For this review, take the finished solid that the model builds, in its own axes (mm). Face numbers are marked on the shaded views. A direction names the side the tool comes from. Coordinates: 2 decimals unless noted, no trailing zeros. Loops run counter-clockwise (first coordinate to the right, second up) from the corner with the lowest first, then second, coordinate; pieces in that order, holes last. Notation, with made-up numbers: (26.5, 60) - (49.5, 60) arc R18 ccw to (49.5, 78) - close; hole circle Ø6 at (33, 27). An arc over 180 degrees is marked (long way). Answer as a JSON object with one key per item and string values. Group by question number.
Item 1: We need section A-A (y = 0). State how many separate pieces and enclosed holes the cut face has, then the cut area to 3 significant figures.
Item 2: We need section B-B (z = -0.5). Give the boundary of the cut face in (x, y).
Item 3: Tool access review of the marked faces 4, 5, 6, 7 and 8: name each direction out of +Z, -Z, +X, -X, +Y, -Y from which nothing blocks a thin tool from reaching the whole face with its end or side.
Item 4: To check wall thickness, follow line 1 (Y direction, x = -49, z = -17.5); line 2 (X direction, y = 4.5, z = -17); line 3 (X direction, y = 4.5, z = -19). State the ranges of each line that lie inside material, in increasing order.
Item 5: Mouldability with a two-part tool opening along X and no side actions: class the marked faces 1, 2 and 3 as released by +X, released by -X, zero draft, split by the parting line, or undercut.
Item 6: Clearance check with flat-ended pins moving along their axes: pin 1 (1.5 mm diameter, centred on x = 30, y = -7, fed in from +Z); pin 2 (2 mm diameter, centred on y = 7.5, z = 1.5, fed in from +X); pin 3 (14 mm diameter, centred on x = 0, z = 26.14, fed in from +Y); pin 4 (8 mm diameter, centred on x = 46.67, y = 0, fed in from -Z). State where each tip first meets the part, or that it passes through.
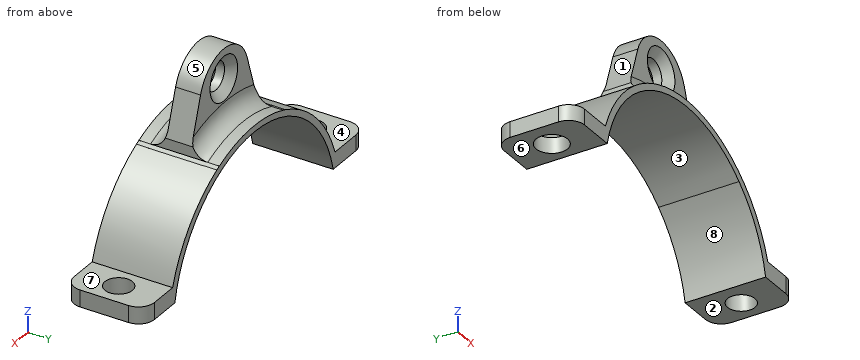
from build123d import *

# Parameters (mm, degrees)
F1_DEPTH  = 3.943235
F3_DEPTH  = 12.7
F4_R      = 5.08
F6_DEPTH  = 12.7
F7_W      = 17.78
F7_H      = 5.3086
F8_DEPTH  = 12.7
F9_DEPTH  = 8.66714
F10_DEPTH = 9.47498
F12_DEPTH = 12.7
F13_DEPTH = 12.7
F14_R     = 4.3985303862
F15_DEPTH = 53.72973
F16_SIZE  = 2.54
F17_SIZE  = 2.54
F18_R     = 5.08
F19_R     = 4.960906564
F19_R_2   = 4.3415616657
F20_DEPTH = 23.4886
F22_DEPTH = 18.208115
F24_DEPTH = 12.7
F26_DEPTH = 20.13737


with BuildPart() as f1:
    # F0 (on Front) → F1 (new body, symmetric)
    with BuildSketch(Plane.XZ):
        with BuildLine():
            Line((-11.7292143404, 26.9492678344), (-17.5938215107, 9.0761780739))
            ThreePointArc((-17.5938215107, 9.0761780739), (0, 11.6662775846), (17.5938215107, 9.0761780739))
            Line((17.5938215107, 9.0761780739), (11.7292143404, 26.9492678344))
            ThreePointArc((11.7292143404, 26.9492678344), (0, 35.4451148535), (-11.7292143404, 26.9492678344))
        make_face()
    extrude(amount=F1_DEPTH, both=True)

    # F2 (on Front) → F3 (join, symmetric)
    with BuildSketch(Plane.XZ):
        with BuildLine():
            Line((36.3047122955, -16.6163872927), (39.93518278, -16.6163872927))
            ThreePointArc((39.93518278, -16.6163872927), (-0.7137528874, 13.5858944169), (-42.1693213284, -15.4993189499))
            Line((-42.1693213284, -15.4993189499), (-39.0973836184, -15.7785862684))
            ThreePointArc((-39.0973836184, -15.7785862684), (-1.101821027, 10.3088316272), (36.3047122955, -16.6163872927))
        make_face()
    extrude(amount=F3_DEPTH, both=True)

    # F4
    f4_edges = [f1.edges().sort_by_distance(p)[0] for p in [
        (0.356921, -3.943235, 13.558065),
        (0.356921, 3.943235, 13.558065),
    ]]
    fillet(f4_edges, radius=F4_R)

    # F5 (on Front) → F6 (join, symmetric)
    with BuildSketch(Plane.XZ):
        Polygon((-39.8543514311, -20.1193168759), (-39.659883827, -15.2054578066), (-57.6343514311, -15.2054578066), (-57.6343514311, -20.1193168759), align=None)
    extrude(amount=F6_DEPTH, both=True)

    # F7 (on Front) → F8 (join, symmetric)
    with BuildSketch(Plane.XZ):
        with Locations((45.0512229579, -18.7627813943)):
            Rectangle(F7_W, F7_H)
    extrude(amount=F8_DEPTH, both=True)

    # F5 (on Front) → F9 (join)
    with BuildSketch(Plane.XZ):
        Polygon((-39.8543514311, -20.1193168759), (-39.659883827, -15.2054578066), (-57.6343514311, -15.2054578066), (-57.6343514311, -20.1193168759), align=None)
    extrude(amount=F9_DEPTH)

    # F7 (on Front) → F10 (join)
    with BuildSketch(Plane.XZ):
        with Locations((45.0512229579, -18.7627813943)):
            Rectangle(F7_W, F7_H)
    extrude(amount=F10_DEPTH)

    # F11 (on Front) → F12 (cut, symmetric)
    with BuildSketch(Plane.XZ):
        with BuildLine():
            ThreePointArc((-40.8051013947, -20.0025010854), (-1.7400987678, -54.2430909447), (38.6715009809, -21.6027013958))
            ThreePointArc((38.6715009809, -21.6027013958), (-0.4185114947, 11.3957328504), (-40.8051013947, -20.0025010854))
        make_face()
    extrude(amount=F12_DEPTH, both=True, mode=Mode.SUBTRACT)

    # F11 (on Front) → F13 (cut, symmetric)
    with BuildSketch(Plane.XZ):
        with BuildLine():
            ThreePointArc((-40.8051013947, -20.0025010854), (-1.7400987678, -54.2430909447), (38.6715009809, -21.6027013958))
            ThreePointArc((38.6715009809, -21.6027013958), (-0.4185114947, 11.3957328504), (-40.8051013947, -20.0025010854))
        make_face()
    extrude(amount=F13_DEPTH, both=True, mode=Mode.SUBTRACT)

    # F14 (on face) → F15 (cut, symmetric)
    with BuildSketch(Plane.XZ.offset(3.943235)):
        with Locations((0, 26.1365994811)):
            Circle(F14_R)
    extrude(amount=F15_DEPTH, both=True, mode=Mode.SUBTRACT)

    # F16
    f16_edges = [f1.edges().sort_by_distance(p)[0] for p in [
        (-4.39853, -3.943235, 26.136599),
    ]]
    chamfer(f16_edges, length=F16_SIZE)

    # F17
    f17_edges = [f1.edges().sort_by_distance(p)[0] for p in [
        (-4.39853, 3.943235, 26.136599),
    ]]
    chamfer(f17_edges, length=F17_SIZE)

    # F18
    f18_edges = [f1.edges().sort_by_distance(p)[0] for p in [
        (53.941223, 12.7, -18.762781),
        (53.941223, -12.7, -18.762781),
        (-57.634351, 12.7, -17.662387),
        (-57.634351, -12.7, -17.662387),
    ]]
    fillet(f18_edges, radius=F18_R)

    # F19 (on face) → F20 (cut)
    with BuildSketch(Plane.XY.offset(-15.2054578066)):
        with Locations((-48.8061010838, 0)):
            Circle(F19_R)
        with Locations((46.67250067, 0)):
            Circle(F19_R_2)
    extrude(amount=-F20_DEPTH, mode=Mode.SUBTRACT)

    # F21 (on Front) → F22 (cut, symmetric)
    with BuildSketch(Plane.XZ):
        with BuildLine():
            Line((-41.792165488, -23.9205155522), (39.0426814556, -25.9368028492))
            ThreePointArc((39.0426814556, -25.9368028492), (-0.4636625416, 11.5973705937), (-41.792165488, -23.9205155522))
        make_face()
    extrude(amount=F22_DEPTH, both=True, mode=Mode.SUBTRACT)

    # F23 (on Front) → F24 (cut, symmetric)
    with BuildSketch(Plane.XZ):
        Polygon((-17.0922335237, 10.6045696884), (-15.9068014473, 11.0168391839), (-15.9068014473, 14.8834753782), align=None)
    extrude(amount=F24_DEPTH, both=True, mode=Mode.SUBTRACT)

    # F25 (on Front) → F26 (cut, symmetric)
    with BuildSketch(Plane.XZ):
        Polygon((17.5980012864, 9.2452950776), (16.2439439446, 13.5627323762), (16.2439439446, 9.859982878), align=None)
    extrude(amount=F26_DEPTH, both=True, mode=Mode.SUBTRACT)


solid = f1.part
Check sheet entries:
{
 "1": {"separate pieces": "3", "enclosed holes": "1", "area": "784 mm2"},
 "2": {"outline": "(-33.24, -12.7) - (-30.42, -12.7) - (-30.42, 12.7) - (-33.24, 12.7) - close; (27.5, -12.7) - (30.64, -12.7) - (30.64, 12.7) - (27.5, 12.7) - close"},
 "3": {"face 4": "+Z, -X, +Y, -Y", "face 5": "+Z, +Y, -Y", "face 6": "-Z, -X, +Y, -Y", "face 7": "+Z, +X, +Y, -Y", "face 8": "-Z, +Y, -Y"},
 "4": {"line 1": "y = -12.7 to -4.96, 4.96 to 12.7", "line 2": "x = -57.63 to -50.89, -46.72 to -40.29, 37.51 to 53.94", "line 3": "x = -57.63 to -50.89, -46.72 to -40.86, 38.09 to 53.94"},
 "5": {"face 1": "released by -X", "face 2": "zero draft", "face 3": "undercut"},
 "6": {"pin 1": "stops at z = 0.95", "pin 2": "stops at x = 29.7", "pin 3": "stops at y = 3.94", "pin 4": "passes through"}
}
